```python
from build123d import *

# Parameters (mm, degrees)
SKETCH1_W           = 38.1
SKETCH1_H           = 21.209
BOSS_EXTRUDE1_DEPTH = 6.35
SKETCH2_R           = 2.667
CUT_EXTRUDE1_DEPTH  = 9.525
CUT_EXTRUDE2_DEPTH  = 9.525
CUT_EXTRUDE4_DEPTH  = 9.525
FILLET2_R           = 3.048


with BuildPart() as part:
    # Sketch1 → Boss-Extrude1 (new body)
    with BuildSketch(Plane(origin=(0, 0, 0), x_dir=(1, 0, 0), z_dir=(0, 1, 0))):
        Rectangle(SKETCH1_W, SKETCH1_H)
    extrude(amount=BOSS_EXTRUDE1_DEPTH)

    # Sketch2 → Cut-Extrude1 (cut)
    with BuildSketch(Plane(origin=(0, 6.35, 0), x_dir=(1, 0, 0), z_dir=(0, 1, 0))):
        with Locations((-12.7, 0)):
            Circle(SKETCH2_R)
        with Locations((12.7, 0)):
            Circle(SKETCH2_R)
    extrude(amount=-CUT_EXTRUDE1_DEPTH, mode=Mode.SUBTRACT)

    # Sketch3 → Cut-Extrude2 (cut)
    with BuildSketch(Plane(origin=(0, 6.35, 0), x_dir=(1, 0, 0), z_dir=(0, 1, 0))):
        Polygon((-19.05, 10.6045), (-15.875, 10.6045), (-19.05, 7.4295), align=None)
        Polygon((19.05, 10.6045), (15.748, 10.6045), (19.05, 7.3025), align=None)
        Polygon((19.05, -10.6045), (15.748, -10.6045), (19.05, -7.3025), align=None)
        Polygon((-19.05, -10.6045), (-15.875, -10.6045), (-19.05, -7.4295), align=None)
    extrude(amount=-CUT_EXTRUDE2_DEPTH, mode=Mode.SUBTRACT)

    # Sketch4 → Cut-Extrude4 (cut)
    with BuildSketch(Plane(origin=(0, 6.35, 0), x_dir=(1, 0, 0), z_dir=(0, 1, 0))):
        Polygon((-19.05, -7.4295), (-15.875, -10.6045), (-15.875, -6.35), (-19.05, -6.35), align=None)
        Polygon((15.748, -10.6045), (19.05, -7.3025), (19.05, -6.35), (-15.875, -6.35), (-15.875, -10.6045), align=None)
    extrude(amount=-CUT_EXTRUDE4_DEPTH, mode=Mode.SUBTRACT)

    # Fillet2
    fillet2_edges = [part.edges().sort_by_distance(p)[0] for p in [
        (-19.05, 3.175, 6.35),
        (19.05, 3.175, 6.35),
    ]]
    fillet(fillet2_edges, radius=FILLET2_R)


solid = part.part
```
Build history of the part. All positions in model axes, mm. Give positions to 0.01 mm unless a question says otherwise; leave off trailing zeros. Order: outer loops, then holes, each group sorted by start corner. A loop starts at its lowest first (then second) coordinate and runs counter-clockwise, first axis right, second up. Notation, with made-up numbers: M 54.25,4.5 L 70.25,4.5 A16 ccw 70.25,24.5 Z; hole C 56.5,-38.75 d2. An arc over 180 degrees is marked long. Write item = value, one per line. Start each with the question number.
(1) Slice it at A-A on y = 0.75. State how many separate pieces and enclosed holes the cut face has, plus the area to 3 significant figures.
(2) Two-plate mould, pull along X, no slides. Class faces 1 (the cylindrical face through (15.244, 3.219, -0.801)), 2 (the cylindrical face through (18.133, 3.131, 5.481)), 3 (the cylindrical face through (-18.181, 3.131, 5.433)), 4 (the flat face through (0, 3, -10.604)): released by +X, released by -X, zero draft, split by the parting line, or undercut.
(3) Slice it at C-C on z = 0. Write the cut outline in (x, y).
(4) Slice it at B-B on x = 12.7. Write the cut outline in (y, z), plus the area to 3 significant figures.
(5) Probe L1, parallel to X at y = 4.5, z = 0; L2, parallel to Z at x = 12.7, y = 2.25. List the from-to ranges inside material, lowest first. Write a range as [from, to].
(6) Slice it at D-D on x = -11. Write the cut outline in (y, z), plus the area to 3 significant figures.
Responses:
q1.separate_pieces = 1
q1.enclosed_holes = 2
q1.area = 587 mm2
q2.face_1 = undercut
q2.face_2 = released by +X
q2.face_3 = released by -X
q2.face_4 = zero draft
q3.outline = M -19.05,0 L -15.37,0 L -15.37,6.35 L -19.05,6.35 Z; M -10.03,0 L 10.03,0 L 10.03,6.35 L -10.03,6.35 Z; M 15.37,0 L 19.05,0 L 19.05,6.35 L 15.37,6.35 Z
q4.outline = M 0,-10.6 L 6.35,-10.6 L 6.35,-2.67 L 0,-2.67 Z; M 0,2.67 L 6.35,2.67 L 6.35,6.35 L 0,6.35 Z
q4.area = 73.8 mm2
q5.L1 = [-19.05, -15.37], [-10.03, 10.03], [15.37, 19.05]
q5.L2 = [-10.6, -2.67], [2.67, 6.35]
q6.outline = M 0,-10.6 L 6.35,-10.6 L 6.35,-2.05 L 0,-2.05 Z; M 0,2.05 L 6.35,2.05 L 6.35,6.35 L 0,6.35 Z
q6.area = 81.6 mm2
